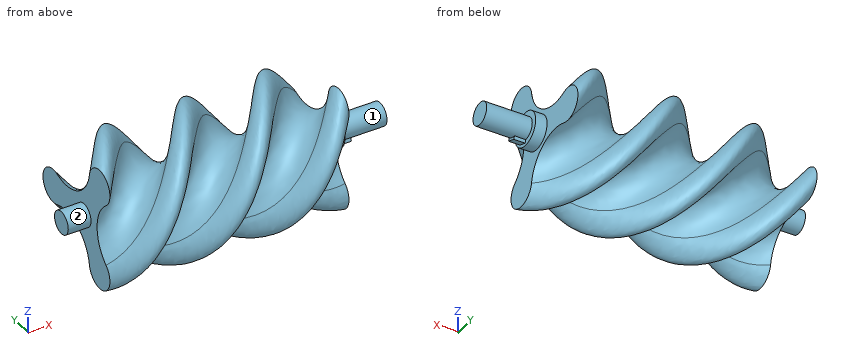
```python
from build123d import *

# Parameters (mm, degrees)
SWEEP1_PITCH             = 210
SWEEP1_HEIGHT            = 210
SWEEP1_RADIUS            = 60
SWEEP1_START_ANGLE       = -90
BOSS_EXTRUDE1_DEPTH      = 50
BOSS_EXTRUDE1_DEPTH_BACK = 230
SKETCH3_R                = 10
SKETCH4_R                = 15
BOSS_EXTRUDE2_DEPTH      = 10
BOSS_EXTRUDE3_DEPTH      = 10


with BuildPart() as part:
    # Sweep1: sweep along a helix
    with BuildLine() as sweep1_path:
        add(Helix(SWEEP1_PITCH, SWEEP1_HEIGHT, SWEEP1_RADIUS, center=(0, 0, 0), direction=(1, 0, 0), lefthand=True, mode=Mode.PRIVATE).rotate(Axis((0, 0, 0), (1, 0, 0)), SWEEP1_START_ANGLE))
    # Sketch1 → Sweep1 (sweep)
    with BuildSketch(Plane(origin=(0, 0, 0), x_dir=(0, 0, -1), z_dir=(1, 0, 0))):
        with BuildLine():
            ThreePointArc((13.984121881, 39.573736532), (0, 60), (-13.984121881, 39.573736532))
            ThreePointArc((-13.984121881, 39.573736532), (-16.30285047, 9.412455108), (-41.2639221, -7.676263468))
            ThreePointArc((-41.2639221, -7.676263468), (-51.961524227, -30), (-27.279800219, -31.897473065))
            ThreePointArc((-27.279800219, -31.897473065), (0, -18.824910215), (27.279800219, -31.897473065))
            ThreePointArc((27.279800219, -31.897473065), (51.961524227, -30), (41.2639221, -7.676263468))
            ThreePointArc((41.2639221, -7.676263468), (16.30285047, 9.412455108), (13.984121881, 39.573736532))
        make_face()
    sweep(path=sweep1_path.line, is_frenet=True)

    # Sketch3 → Boss-Extrude1 (add, two sides: drawn at the far end of the back side and taken through both)
    with BuildSketch(Plane(origin=(210, 0, 0), x_dir=(0, 0, -1), z_dir=(1, 0, 0)).offset(-BOSS_EXTRUDE1_DEPTH_BACK)):
        Circle(SKETCH3_R)
    extrude(amount=BOSS_EXTRUDE1_DEPTH + BOSS_EXTRUDE1_DEPTH_BACK)

    # Sketch4 → Boss-Extrude2 (add)
    with BuildSketch(Plane(origin=(210, 0, 0), x_dir=(0, 0, -1), z_dir=(1, 0, 0))):
        Circle(SKETCH4_R)
    extrude(amount=BOSS_EXTRUDE2_DEPTH)

    # Sketch5 → Boss-Extrude3 (add)
    with BuildSketch(Plane(origin=(220, 0, 0), x_dir=(0, 0, -1), z_dir=(1, 0, 0))):
        Polygon((6.066543677, 2.048669767), (12.644392023, -0.345471237), (9.908230876, -7.863012203), (3.330382531, -5.4688712), align=None)
    extrude(amount=BOSS_EXTRUDE3_DEPTH)


solid = part.part
```
Can you work these out from the model? Positions are in its coordinate system, mm. Face numbers are marked on the shaded views. A direction names the side the tool comes from. Give positions to 0.01 mm unless a question says otherwise; leave off trailing zeros. Use a Markdown table: item, result. Add a question column.
Q1. On a 3-axis mill with a long thin cutter (end or side, diameter ignored), from which of +Z, -Z, +X, -X, +Y, -Y can I reach the whole of each face in a straight line? I mean the marked faces 1 and 2. Say none if no direction works.
Q2. I'm going to push flat-ended pins straight in: pin 1 (2 mm diameter, centred on y = -17, z = 48, fed in from -X); pin 2 (6 mm diameter, centred on x = 126, y = 39, fed in from -Z); pin 3 (10 mm diameter, centred on x = 154.5, y = -33.5, fed in from +Z). Where does each tip first touch, or does it pass through?
Q3. If we section it at A-A on z = -30.5: Count the separate pieces of the cut face and the enclosed holes in it, plus the area to 3 significant figures.
Q4. Please list where these lines run through material, in increasing order: line 1 along X through (y, z) = (50, 22.5); line 2 along X through (y, z) = (-35, 43); line 3 along X through (y, z) = (-38.5, -5.5).
Answers follow:
| question | item | result |
|---|---|---|
| 1 | face 1 | +X |
| 1 | face 2 | -X |
| 2 | pin 1 | stops at x = 0 |
| 2 | pin 2 | stops at z = -0.45 |
| 2 | pin 3 | stops at z = -3.08 |
| 3 | separate pieces | 4 |
| 3 | enclosed holes | 0 |
| 3 | area | 6,640 mm^2 |
| 4 | line 1 | x = 48.23 to 63.51, 118.23 to 133.51, 188.23 to 203.51 |
| 4 | line 2 | x = 0 to 1.88, 57.45 to 71.88, 127.45 to 141.88, 197.45 to 210 |
| 4 | line 3 | x = 18.87 to 41.65, 88.87 to 111.65, 158.87 to 181.65 |
